Part print with two shaded views. Sizes in mm from the minimum x, y, z corner. Give positions to 0.01 mm unless a question says otherwise; leave off trailing zeros. Write each loop counter-clockwise with the first axis right and the second up, starting at its lowest first coordinate (ties: lowest second). Pieces come first, ordered by that corner, then holes.
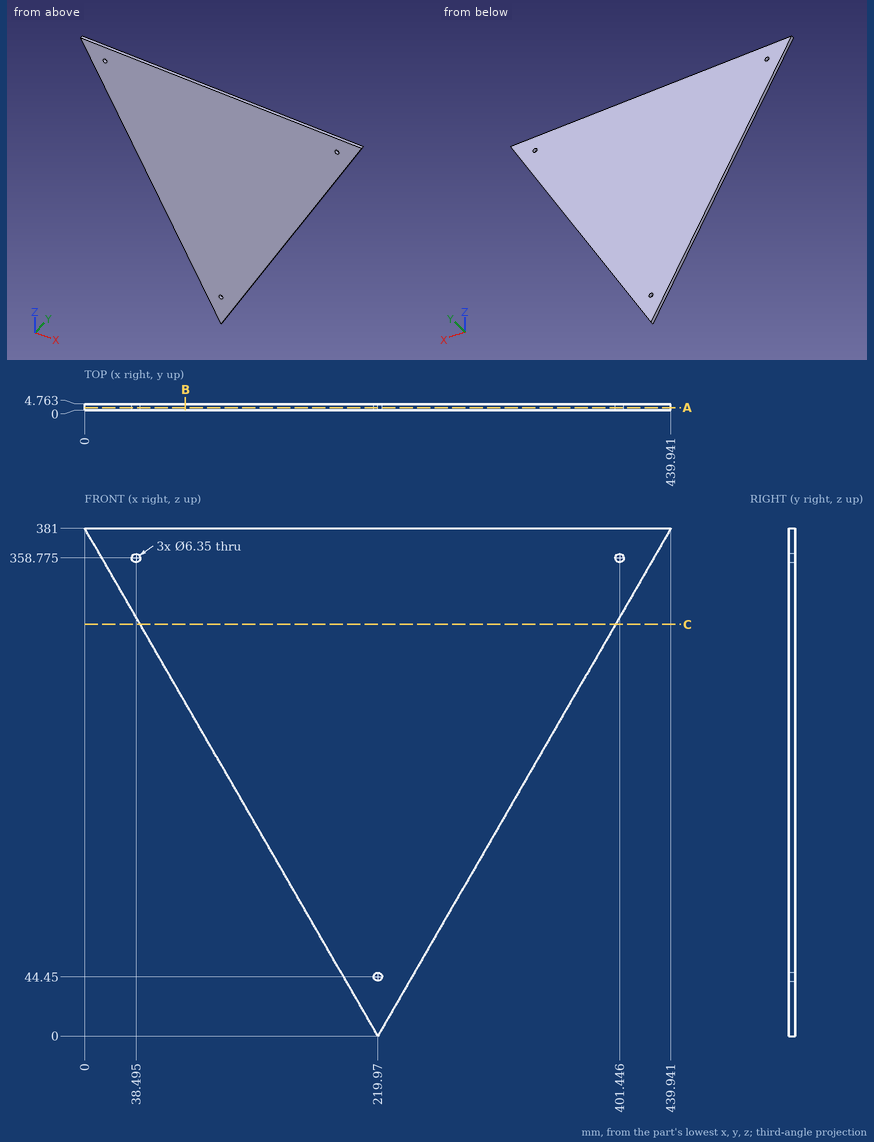
1) Flat gauge pin, fed straight in: P1, Ø4, axis at x = 38.49, z = 358.78, coming from the +Y side. Where does the tip first touch, or does it go through?
Check result:
P1: passes through
2) Saw through at B-B (x = 75.5). Write the cut outline in (y, z), and give its area (3 significant figures).
Check result:
outline: (0, 250.23) - (4.76, 250.23) - (4.76, 381) - (0, 381) - close
area: 623 mm2
3) Saw through at A-A (y = 2). State how many separate pieces and enclosed holes the cut face has, and give its area (3 significant figures).
Check result:
separate pieces: 1
enclosed holes: 3
area: 83,700 mm2
4) Drill centre lines: L1, parallel to X at y = 2.8, z = 44.45 (1 decimal); L2, parallel to Z at x = 219.5, y = 4.1 (1 decimal); L3, parallel to Z at x = 338, y = 2.4 (1 decimal). Where is each one in solid material? Low to high.
Check result:
L1: x = 194.3 to 216.8, 223.1 to 245.6
L2: z = 0.8 to 41.3, 47.6 to 381
L3: z = 204.4 to 381
5) Saw through at C-C (z = 309). Write the cut outline in (x, y).
Check result:
outline: (41.57, 0) - (398.37, 0) - (398.37, 4.76) - (41.57, 4.76) - close
